from build123d import *

# Parameters (mm, degrees)
ESQUISSE2_R             = 2.5
BOSS_EXTRU_1_DEPTH      = 6
ESQUISSE3_R             = 1.25
ENL_V_MAT_EXTRU_1_DEPTH = 14.3
ESQUISSE4_R             = 9
ENL_V_MAT_EXTRU_2_DEPTH = 5
ESQUISSE6_R             = 9
ESQUISSE6_R_2           = 7


with BuildPart() as part:
    # Esquisse1 → Base-Révolution (revolve)
    with BuildSketch(Plane.XY, mode=Mode.PRIVATE) as base_r_volution_sk:
        Polygon((2, 16.5), (38, 16.5), (38, 18.5), (40, 18.5), (40, 0), (38, 0), (38, 15.5), (2, 15.5), (2, 0), (0, 0), (0, 18.5), (2, 18.5), align=None)
    revolve(base_r_volution_sk.sketch.rotate(Axis((-25.081544634, 0, 0), (1, 0, 0)), 90), axis=Axis((-25.081544634, 0, 0), (1, 0, 0)))

    # Esquisse2 → Boss.-Extru.1 (add)
    with BuildSketch(Plane(origin=(40, 0, 0), x_dir=(0, 0, -1), z_dir=(1, 0, 0))):
        with Locations(Location((0, 13.61181584, 0), (0, 0, 180))):
            Circle(ESQUISSE2_R)
    extrude(amount=BOSS_EXTRU_1_DEPTH)

    # Esquisse3 → Enlèv. mat.-Extru.1 (cut)
    with BuildSketch(Plane(origin=(46, 0, 0), x_dir=(0, 0, -1), z_dir=(1, 0, 0))):
        with Locations((0, 13.61181584)):
            Circle(ESQUISSE3_R)
    extrude(amount=-ENL_V_MAT_EXTRU_1_DEPTH, mode=Mode.SUBTRACT)

    # Esquisse4 → Enlèv. mat.-Extru.2 (cut)
    with BuildSketch(Plane.ZY):
        Circle(ESQUISSE4_R)
    extrude(amount=-ENL_V_MAT_EXTRU_2_DEPTH, mode=Mode.SUBTRACT)

    # Boss.-Balayage1: sweep along a path in Esquisse7
    with BuildLine(Plane.XY) as boss_balayage1_path:
        Line((2, 0), (-2, 0))
        ThreePointArc((-2, 0), (-23.213203436, -8.786796564), (-32, -30))
    # Esquisse6 → Boss.-Balayage1 (sweep)
    with BuildSketch(Plane(origin=(2, 0, 0), x_dir=(0, 0, -1), z_dir=(1, 0, 0))):
        Circle(ESQUISSE6_R)
        Circle(ESQUISSE6_R_2, mode=Mode.SUBTRACT)
    sweep(path=boss_balayage1_path.line)


solid = part.part
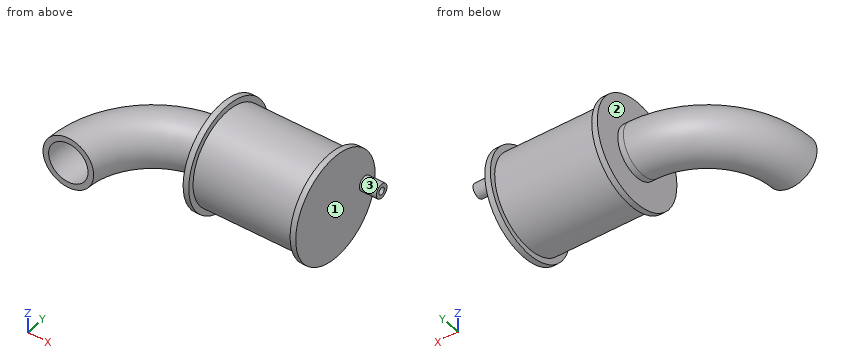
Geometry: final body of the model. Coordinates: model frame, mm. Face numbers are marked on the shaded views. Give positions to 0.01 mm unless a question says otherwise; leave off trailing zeros. Return JSON: item names as keys, results as strings. Group by question number.
1) Mould query, pull axis X, two halves, no side actions, for the marked faces 1, 2 and 3. Classes: released by +X, released by -X, zero draft, split by the parting line, or undercut.
2) First-contact query: P1, Ø12, axis at x = -19, z = -13.5, coming from the +Y side; P2, Ø4, axis at y = 9, z = -2.5, coming from the +X side; P3, Ø6, axis at x = -1, y = -9.5, coming from the -Z side. Flat tips, straight axial feed; report the tip coordinate or a pass-through.
3) Section A-A on y = -10. State how many separate pieces and enclosed holes the cut face has, plus the area to 3 significant figures.
4) Line query: line 1 (Y direction, x = 43, z = 0); line 2 (X direction, y = 14, z = 9); line 3 (Z direction, x = -22.5, y = -7.5). Output: solid intervals per line, ascending.
Filled in:
{
 "1": {"face 1": "released by +X", "face 2": "undercut", "face 3": "zero draft"},
 "2": {"P1": "stops at y = 1.02", "P2": "stops at x = 40", "P3": "stops at z = -17.26"},
 "3": {"separate pieces": "2", "enclosed holes": "2", "area": "371 mm^2"},
 "4": {"line 1": "y = 11.11 to 12.36, 14.86 to 16.11", "line 2": "x = 0 to 2, 38 to 40", "line 3": "z = -8.99 to -6.99, 6.99 to 8.99"}
}
